Check sheet for the modelled part. Datum: model origin and axes. Units: mm. Face numbers are marked on the shaded views. A direction names the side the tool comes from. Round coordinates to 2 decimals unless told otherwise and drop trailing zeros. Write each loop counter-clockwise with the first axis right and the second up, starting at its lowest first coordinate (ties: lowest second). Pieces come first, ordered by that corner, then holes. Notation, with made-up numbers: (-17, -36.75) - (27, -36.75) arc R13 ccw to (27, -29.75) - close; hole circle Ø2 at (-36, 33.5). An arc over 180 degrees is marked (long way). Answer as a JSON object with one key per item and string values. Group by question number.
Item 1: Sectioned sample at D-D on y = -0.5. Record the boundary of the cut face in (x, z), plus the area to 3 significant figures.
Item 2: Release check for a two-part mould opening along Y. For the marked faces 1, 2 and 3 record: pulls with the +Y half, pulls with the -Y half, needs draft (parallel to the pull), parting line crosses it, or undercut.
Item 3: Set-up check for the marked faces 4 and 5: record each of +Z, -Z, +X, -X, +Y, -Y from which the full face is reachable in a straight line by a thin tool's end or side.
Item 4: Sectioned sample at A-A on z = 3.5. Record the boundary of the cut face in (x, y).
Item 5: Sectioned sample at B-B on x = 0. Record the boundary of the cut face in (y, z).
Item 6: Gauge pin test, flat ends, axial feed: P1, Ø0.8, axis at x = 0, z = -6.5, coming from the -Y side; P2, Ø1.5, axis at y = 4, z = 5, coming from the -X side; P3, Ø6, axis at y = -1, z = 5.5, coming from the +X side; P4, Ø5, axis at x = 0, y = -0.5, coming from the -Z side. Record the tip position at first contact, or that the pin passes through.
Item 7: Thickness scan on line 1 (Y direction, x = 0, z = 5); line 2 (Z direction, x = 0, y = 4.7); line 3 (Y direction, x = -1, z = -8). Record the ranges inside material, lowest first.
Item 8: Sectioned sample at C-C on z = -6.5. Record the boundary of the cut face in (x, y).
Autodesk Inventor part; units mm, degrees
ref_plane "YZ Plane" through (0, 0, 0) normal (1, 0, 0) x (0, 1, 0)
ref_plane "XZ Plane" through (0, 0, 0) normal (0, 1, 0) x (-1, 0, 0)
ref_plane "XY Plane" through (0, 0, 0) normal (0, 0, 1) x (1, 0, 0)
sketch "Sketch1" plane through (0, 0, 0) normal (0, 0, 1) x (1, 0, 0)
  circle A0 centre (0, 0) radius 2.75
  line L0 (0, 0) -> (3.1, 0) construction
  line L1 (0, 0) -> (1.55, 2.6847) construction
  line L2 (0, 0) -> (-1.55, 2.6847) construction
  line L3 (0, 0) -> (-3.1, 0) construction
  line L4 (0, 0) -> (-1.55, -2.6847) construction
  line L5 (0, 0) -> (1.55, -2.6847) construction
  line L6 (-1.55, 2.6847) -> (1.55, 2.6847) construction
  line L7 (1.55, 2.6847) -> (3.1, 0) construction
  line L8 (3.1, 0) -> (1.55, -2.6847) construction
  line L9 (1.55, -2.6847) -> (-1.55, -2.6847) construction
  line L10 (-1.55, -2.6847) -> (-3.1, 0) construction
  line L11 (-3.1, 0) -> (-1.55, 2.6847) construction
  line L12 (3.5619, 0) -> (1.7809, 3.0847)
  line L13 (1.7809, 3.0847) -> (-1.7809, 3.0847)
  line L14 (-1.7809, 3.0847) -> (-3.5619, 0)
  line L15 (-3.5619, 0) -> (-1.7809, -3.0847)
  line L16 (-1.7809, -3.0847) -> (1.7809, -3.0847)
  line L17 (1.7809, -3.0847) -> (3.5619, 0)
  line L18 (3.2243, 5.5847) -> (6.4486, 0)
  line L19 (6.4486, 0) -> (3.2243, -5.5847)
  line L20 (3.2243, -5.5847) -> (-3.2243, -5.5847)
  line L21 (-3.2243, -5.5847) -> (-6.4486, 0)
  line L22 (-6.4486, 0) -> (-3.2243, 5.5847)
  line L23 (-3.2243, 5.5847) -> (3.2243, 5.5847)
  dimension "d0" = 5.5
  dimension "d2" = 3.1
  dimension "d5" = 360
  dimension "d7" = 0.4
  dimension "d8" = 2.5
extrude "Extrusion1" add sketch "Sketch1" along normal blind 8 contours L17 L16 L15 L14 L13 L12 | L18 L19 L20 L21 L22 L23
extrude "Extrusion2" add sketch "Sketch1" against normal blind 10 contours L18 L19 L20 L21 L22 L23
sketch "Sketch2" plane through (-3.2243, 5.5847, 8) normal (0, 1, 0) x (1, 0, 0)
  line L0 (0, 0) -> (0, 18)
  line L1 (0, 8) -> (6.4486, 8)
  line L2 (3.2243, 8) -> (3.2243, 18) construction
  line L3 (6.4486, 18) -> (0, 18)
  line L4 (6.4486, 18) -> (6.4486, 0)
  circle A0 centre (3.2243, 14.5) radius 0.65
  dimension "d13" = 1.3
  dimension "d14" = 6.5
extrude "Extrusion3" cut sketch "Sketch2" against normal blind 15 contours A0
properties part number "Acople_Motor_"
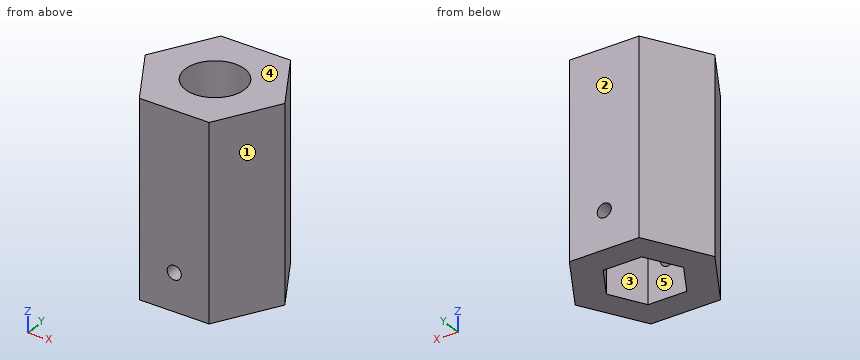
Completed:
{
 "1": {"outline": "(-6.16, -10) - (-3.27, -10) - (-3.27, 0) - (-2.7, 0) - (-2.7, 8) - (-6.16, 8) - close; (2.7, 0) - (3.27, 0) - (3.27, -10) - (6.16, -10) - (6.16, 8) - (2.7, 8) - close", "area": "113 mm²"},
 "2": {"face 1": "pulls with the -Y half", "face 2": "pulls with the +Y half", "face 3": "undercut"},
 "3": {"face 4": "+Z, +X, -X, +Y, -Y", "face 5": "-Z"},
 "4": {"outline": "(-6.45, 0) - (-3.22, -5.58) - (3.22, -5.58) - (6.45, 0) - (3.22, 5.58) - (-3.22, 5.58) - close; hole circle Ø5.5 at (0, 0)"},
 "5": {"outline": "(-5.58, -10) - (-3.08, -10) - (-3.08, -7.15) - (-5.58, -7.15) - close; (-5.58, -5.85) - (-3.08, -5.85) - (-3.08, 0) - (-2.75, 0) - (-2.75, 8) - (-5.58, 8) - close; (2.75, 0) - (3.08, 0) - (3.08, -5.85) - (5.58, -5.85) - (5.58, 8) - (2.75, 8) - close; (3.08, -10) - (5.58, -10) - (5.58, -7.15) - (3.08, -7.15) - close"},
 "6": {"P1": "through", "P2": "x = -4.57", "P3": "x = 6.45", "P4": "z = 0"},
 "7": {"line 1": "-5.58 to -2.75, 2.75 to 5.58", "line 2": "-10 to -7.15, -5.85 to 8", "line 3": "-5.58 to -3.08, 3.08 to 5.58"},
 "8": {"outline": "(-6.45, 0) - (-3.22, -5.58) - (-0.65, -5.58) - (-0.65, -3.08) - (-1.78, -3.08) - (-3.56, 0) - (-1.78, 3.08) - (-0.65, 3.08) - (-0.65, 5.58) - (-3.22, 5.58) - close; (0.65, -5.58) - (3.22, -5.58) - (6.45, 0) - (3.22, 5.58) - (0.65, 5.58) - (0.65, 3.08) - (1.78, 3.08) - (3.56, 0) - (1.78, -3.08) - (0.65, -3.08) - close"}
}
